Read the model definition and answer for the solid it produces. Units are mm, in the model's axes. A direction names the side the tool comes from. Give positions to 0.01 mm unless a question says otherwise; leave off trailing zeros. Write each loop counter-clockwise with the first axis right and the second up, starting at its lowest first coordinate (ties: lowest second). Pieces come first, ordered by that corner, then holes. Notation, with made-up numbers: (-29, 72.5) -> (-4, 72.5) arc R11 cw to (-4, 77.5) -> close; hole circle Ø8 at (-9.75, 4). An arc over 180 degrees is marked (long way). Use a Markdown table: item, result.
from build123d import *

# Parameters (mm, degrees)
SKETCH_1_W          = 70
SKETCH_1_H          = 16
EXTRUDE_1_DEPTH     = 8
SKETCH_2_W          = 50
SKETCH_2_H          = 8
CUT_EXTRUDE_1_DEPTH = 37.783148315
SKETCH_3_R          = 1.25
CUT_EXTRUDE_2_DEPTH = 20


with BuildPart() as part:
    # 草图1 → 凸台-拉伸1 (new body)
    with BuildSketch(Plane(origin=(0, 0, 0), x_dir=(1, 0, 0), z_dir=(0, 1, 0))):
        Rectangle(SKETCH_1_W, SKETCH_1_H)
    extrude(amount=EXTRUDE_1_DEPTH)

    # 草图2 → 切除-拉伸1 (cut, through all)
    with BuildSketch(Plane(origin=(0, 8, 0), x_dir=(1, 0, 0), z_dir=(0, 1, 0))):
        with Locations((0, 4)):
            Rectangle(SKETCH_2_W, SKETCH_2_H)
    extrude(amount=-CUT_EXTRUDE_1_DEPTH, mode=Mode.SUBTRACT)

    # 草图3 → 切除-拉伸2 (cut)
    with BuildSketch(Plane(origin=(35, 0, 0), x_dir=(0, 0, -1), z_dir=(1, 0, 0))):
        with Locations((-4, 4)):
            Circle(SKETCH_3_R)
        with Locations((4, 4)):
            Circle(SKETCH_3_R)
    cut_extrude_2 = extrude(amount=-CUT_EXTRUDE_2_DEPTH, mode=Mode.SUBTRACT)

    # 镜向1: 切除-拉伸2 across plane
    add(cut_extrude_2.mirror(Plane(origin=(0, 0, 0), x_dir=(0, 0, 1), z_dir=(1, 0, 0))), mode=Mode.SUBTRACT)


solid = part.part
Item 1: A cutting plane is placed at D-D (z = 4). Give the vertices of the cut face in (x, y).
Return value:
| item | result |
|---|---|
| outline | (-35, 0) -> (35, 0) -> (35, 2.75) -> (15, 2.75) -> (15, 5.25) -> (35, 5.25) -> (35, 8) -> (-35, 8) -> (-35, 5.25) -> (-15, 5.25) -> (-15, 2.75) -> (-35, 2.75) -> close |
Item 2: Straight lines are drawn through the part: line 1 along Y through (x, z) = (-26.75, -4); line 2 along Z through (x, y) = (30.5, 3); line 3 along X through (y, z) = (7.75, -6.5). For each, find the intervals that lie inside material, in ascending order. Write a range as [from, to].
Return value:
| item | result |
|---|---|
| line 1 | [0, 2.75], [5.25, 8] |
| line 2 | [-8, -4.75], [-3.25, 3.25], [4.75, 8] |
| line 3 | [-35, -25], [25, 35] |
Item 3: For a pull along Y with two mould halves and no side action, classify faces 1 (the face through (-15, 4, 4)), 2 (the face through (0, 0, 3)), 3 (the face through (30.07, 2.891, -4.577)), 4 (the face through (35, 4, 0)) as +Y half, -Y half, draft (parallel to the pull), parting line (faces both ways), or undercut.
Return value:
| item | result |
|---|---|
| face 1 | undercut |
| face 2 | -Y half |
| face 3 | undercut |
| face 4 | draft |
Item 4: A tool of negligible diameter and unlimited length cuts with its end or side. For faces 5 (the face through (-35, 4, 0)), 6 (the face through (15, 4, 4)), 7 (the face through (-25.14, 2.78, 4.27)), 8 (the face through (25, 5, -3)), from which of +Z, -Z, +X, -X, +Y, -Y can it reach the whole face along a straight path? Write none if from no direction.
Return value:
| item | result |
|---|---|
| face 5 | +Z, -Z, -X, +Y, -Y |
| face 6 | +X |
| face 7 | -X |
| face 8 | -Z, +Y, -Y |
Item 5: A cutting plane is placed at C-C (z = -4). Give the vertices of the cut face in (x, y).
Return value:
| item | result |
|---|---|
| outline | (-35, 0) -> (-25, 0) -> (-25, 2.75) -> (-35, 2.75) -> close; (-35, 5.25) -> (-25, 5.25) -> (-25, 8) -> (-35, 8) -> close; (25, 0) -> (35, 0) -> (35, 2.75) -> (25, 2.75) -> close; (25, 5.25) -> (35, 5.25) -> (35, 8) -> (25, 8) -> close |
Item 6: A cutting plane is placed at A-A (y = 4). Give the vertices of the cut face in (x, z), then the cut area to 3 significant figures.
Return value:
| item | result |
|---|---|
| outline | (-35, -8) -> (-25, -8) -> (-25, -5.25) -> (-35, -5.25) -> close; (-35, -2.75) -> (-25, -2.75) -> (-25, 0) -> (25, 0) -> (25, -2.75) -> (35, -2.75) -> (35, 2.75) -> (15, 2.75) -> (15, 5.25) -> (35, 5.25) -> (35, 8) -> (-35, 8) -> (-35, 5.25) -> (-15, 5.25) -> (-15, 2.75) -> (-35, 2.75) -> close; (25, -8) -> (35, -8) -> (35, -5.25) -> (25, -5.25) -> close |
| area | 570 mm^2 |
Item 7: This flat-tipped pin is pushed along its axis until it touches: P1, Ø2, axis at x = -19, y = 4.5, coming from the -Z side. Where does it stop, or does it pass through?
Return value:
| item | result |
|---|---|
| P1 | z = 0 |
Item 8: A cutting plane is placed at B-B (x = 31). Give the vertices of the cut face in (y, z).
Return value:
| item | result |
|---|---|
| outline | (0, -8) -> (8, -8) -> (8, 8) -> (0, 8) -> close; hole circle Ø2.5 at (4, -4); hole circle Ø2.5 at (4, 4) |
